For this review, take the finished solid that the model builds, in its own axes (mm). Face numbers are marked on the shaded views. A direction names the side the tool comes from. Round coordinates to 2 decimals unless told otherwise and drop trailing zeros. Write each loop counter-clockwise with the first axis right and the second up, starting at its lowest first coordinate (ties: lowest second). Pieces come first, ordered by that corner, then holes. Notation, with made-up numbers: (-3, -22) -> (38, -22) arc R20 ccw to (38, -7) -> close; hole circle Ø2 at (25, 33.5). An arc over 180 degrees is marked (long way). Answer in a Markdown table with one row per item. Add a question column.
```python
from build123d import *

# Parameters (mm, degrees)
EXTRUDE1_DEPTH     = 11.2014
EXTRUDE2_DEPTH     = 3.000375
CIRPATTERN1_COUNT  = 2
CIRPATTERN1_ANGLE  = 90
SKETCH4_R          = 7.62
CUT_EXTRUDE1_DEPTH = 20.4343
SKETCH7_R          = 1.8161
CUT_EXTRUDE2_DEPTH = 44.301517424


with BuildPart() as part:
    # Sketch1 → Revolve1 (revolve)
    with BuildSketch(Plane.XY, mode=Mode.PRIVATE) as revolve1_sk:
        Polygon((20.4343, 7.62), (20.4343, 8.89), (19.34845, 8.89), (11.7475, 13.335), (11.7475, 10.668), (1.5875, 10.668), (1.5875, 13.97), (-1.5875, 13.97), (-1.5875, 2.8575), (-11.7475, 2.8575), (-11.7475, 3.81), (-17.30375, 2.270125), (-18.0975, 2.270125), (-18.0975, 1.8161), (1.5875, 1.8161), (1.5875, 7.62), align=None)
    revolve(revolve1_sk.sketch.rotate(Axis((0, 0, 0), (1, 0, 0)), 90), axis=Axis((0, 0, 0), (1, 0, 0)))

    # Sketch2 → Revolve2 (revolve)
    with BuildSketch(Plane.XY, mode=Mode.PRIVATE) as revolve2_sk:
        with BuildLine():
            Line((3.39598, 10.668), (1.5875, 10.668))
            Line((1.5875, 10.668), (1.5875, 12.47648))
            ThreePointArc((1.5875, 12.47648), (2.117191528, 11.197691528), (3.39598, 10.668))
        make_face()
        with BuildLine():
            Line((-7.14375, 2.8575), (-1.5875, 2.8575))
            Line((-1.5875, 2.8575), (-1.5875, 8.41375))
            ThreePointArc((-1.5875, 8.41375), (-3.214887947, 4.484887947), (-7.14375, 2.8575))
        make_face()
    revolve(revolve2_sk.sketch.rotate(Axis((0, 0, 0), (1, 0, 0)), 90), axis=Axis((0, 0, 0), (1, 0, 0)))

    # Sketch3 → Extrude1 (add, symmetric)
    with BuildSketch(Plane(origin=(0, 0, 0), x_dir=(-1, 0, 0), z_dir=(0, 0.7071067811865488, 0.7071067811865462))):
        with BuildLine():
            Line((-5.330825, 0.542925), (-9.812655, 0.542925))
            ThreePointArc((-9.812655, 0.542925), (-10.35558, 0), (-9.812655, -0.542925))
            Line((-9.812655, -0.542925), (-5.330825, -0.542925))
            ThreePointArc((-5.330825, -0.542925), (-4.7879, 0), (-5.330825, 0.542925))
        make_face()
    extrude1 = extrude(amount=EXTRUDE1_DEPTH, both=True)

    # Sketch6 → Extrude2 (add, symmetric)
    with BuildSketch(Plane(origin=(0, 0, 0), x_dir=(-1, 0, 0), z_dir=(0, 0.7071067811865488, 0.7071067811865462))):
        with BuildLine():
            Line((8.307916667, 0.396875), (10.583333333, 0.396875))
            ThreePointArc((10.583333333, 0.396875), (10.980208333, 0), (10.583333333, -0.396875))
            Line((10.583333333, -0.396875), (8.307916667, -0.396875))
            ThreePointArc((8.307916667, -0.396875), (7.911041667, 0), (8.307916667, 0.396875))
        make_face()
    extrude2 = extrude(amount=EXTRUDE2_DEPTH, both=True)

    # CirPattern1: Extrude1, Extrude2 ×2 about axis
    cirpattern1_axis = Axis((0, 0, 0), (1, 0, 0))
    add([extrude1.rotate(cirpattern1_axis, i * CIRPATTERN1_ANGLE / (CIRPATTERN1_COUNT - 1)) for i in range(1, CIRPATTERN1_COUNT)])
    add([extrude2.rotate(cirpattern1_axis, i * CIRPATTERN1_ANGLE / (CIRPATTERN1_COUNT - 1)) for i in range(1, CIRPATTERN1_COUNT)])

    # Sketch4 → Cut-Extrude1 (cut)
    with BuildSketch(Plane(origin=(20.4343, 0, 0), x_dir=(0, 0, -1), z_dir=(1, 0, 0))):
        with Locations(Location((0, 0, 0), (0, 0, 180))):
            Circle(SKETCH4_R)
    extrude(amount=-CUT_EXTRUDE1_DEPTH, mode=Mode.SUBTRACT)

    # Sketch7 → Cut-Extrude2 (cut, through all)
    with BuildSketch(Plane.ZY.offset(18.0975)):
        Circle(SKETCH7_R)
    extrude(amount=-CUT_EXTRUDE2_DEPTH, mode=Mode.SUBTRACT)


solid = part.part
```
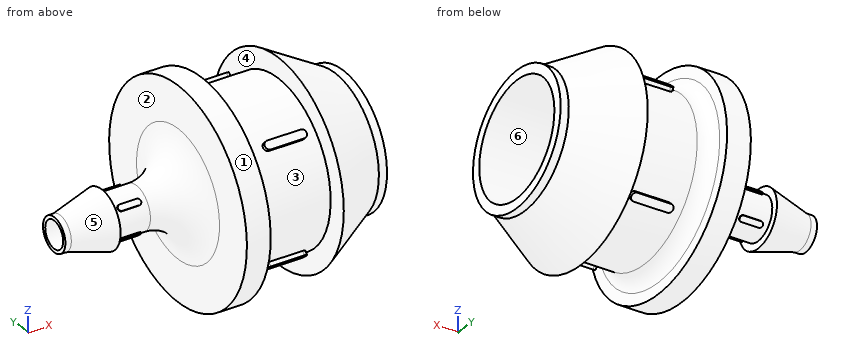
1. For L1, parallel to Y at x = -8, z = 0; L2, parallel to Y at x = 7.5, z = 0; L3, parallel to X at y = 2.75, z = 12.75, list the stretches that pass through material, from the lowest coordinate up. Write a range as [from, to].
2. The part is to be moulded in two halves that separate along Z. For the marked faces 4, 5 and 6, say which applies: pulls with the +Z half, pulls with the -Z half, needs draft (parallel to the pull), parting line crosses it, or undercut.
3. We need section A-A (x = 16). Write out the cut boundary in (y, z), plus the area to 3 significant figures.
4. Tool access review of the marked faces 1, 2 and 3: name each direction out of +Z, -Z, +X, -X, +Y, -Y from which nothing blocks a thin tool from reaching the whole face with its end or side.
5. Clearance check with flat-ended pins moving along their axes: pin 1 Ø5 at (y, z) = (-4, -0.5) entering from +X; pin 2 Ø5 at (y, z) = (9, -0.5) entering from +X; pin 3 Ø4 at (x, y) = (16, 6.5) entering from +Z; pin 4 Ø3 at (x, y) = (0.5, 2.5) entering from -Z. State where each tip first meets the part, or that it passes through.
Response:
| question | item | result |
|---|---|---|
| 1 | L1 | [-2.86, -1.82], [1.82, 2.86] |
| 1 | L2 | [-10.67, -7.62], [7.62, 10.67] |
| 1 | L3 | [-1.59, 1.59], [11.75, 12.25] |
| 2 | face 4 | needs draft |
| 2 | face 5 | parting line crosses it |
| 2 | face 6 | undercut |
| 3 | outline | circle Ø21.7 at (0, 0); hole circle Ø15.24 at (0, 0) |
| 3 | area | 187 mm2 |
| 4 | face 1 | +X, -X |
| 4 | face 2 | -X |
| 4 | face 3 | none |
| 5 | pin 1 | x = 0 |
| 5 | pin 2 | x = 20.43 |
| 5 | pin 3 | z = 10.52 |
| 5 | pin 4 | z = -13.93 |
